Read the model definition and answer for the solid it produces. Units are mm, in the model's axes. A direction names the side the tool comes from. Round coordinates to 2 decimals unless told otherwise and drop trailing zeros. Write each loop counter-clockwise with the first axis right and the second up, starting at its lowest first coordinate (ties: lowest second). Pieces come first, ordered by that corner, then holes. Notation, with made-up numbers: (88, -23) - (122, -23) arc R13 cw to (122, -6) - close; hole circle Ø5 at (71, -34.5). An arc over 180 degrees is marked (long way). One line per item, written item: value. Start each with the question number.
(1) A cutting plane is placed at B-B, the plane y = 13. State how many separate pieces and enclosed holes the cut face has, plus the area to 3 significant figures.
(2) Find the intervals of material crossed by L1, parallel to X at y = 17.25, z = 0; L2, parallel to X at y = 14.25, z = -12; L3, parallel to Z at x = 24.5, y = 8, in increasing order.
(3) A cutting plane is placed at A-A, the plane z = 0. Determine the outline of the cut face in (x, y).
(4) The mould has two halves that part along Z. Classify faces 1 (the face through (-33.907, 11.619, 60.579)), 2 (the face through (-32.51, 11.62, -59.15)), 3 (the face through (35.41, 11, 1)): +Z half, -Z half, draft (parallel to the pull), parting line (faces both ways), or undercut.
(5) Flat-ended cylindrical pins translate along their axes: pin 1 Ø1.5 at (x, z) = (-6.5, 15) entering from +Y; pin 2 Ø8 at (x, y) = (19, 21.5) entering from +Z; pin 3 Ø8 at (x, z) = (0, 0) entering from +Y. Find the tip coordinate at first contact, or state that the pin passes through.
(6) For faces 4 (the face through (-35.41, 11, -1)), 5 (the face through (32.555, 11.619, -59.103)), determine the directions among +Z, -Z, +X, -X, +Y, -Y from which every point of the face is accessible in a straight line to the end or side of a thin tool.
(7) A cutting plane is placed at D-D, the plane x = 20.5. Determine the outline of the cut face in (y, z).
(8) A cutting plane is placed at C-C, the plane z = -44.5. Determine the outline of the cut face in (x, y), plus the area to 3 significant figures.
from build123d import *

# Parameters (mm, degrees)
BASE_EXTRUDE_DEPTH     = 20
FILLET1_R              = 5
FILLET2_R              = 3
SHELL1_T               = -2
RIB1_REACH             = 75.175
SKETCH6_WALLS_W        = 2
SKETCH6_WALLS_H        = 216.25372280356578
FILLET5_RADIUS         = 1
FILLET5_LENGTH         = 120.01036485
SKETCH3_R              = 10
CYLBOSS_DEPTH          = 25
FILLET4_R              = 1
COUNTERSNK_D           = 5
COUNTERSNK_CSINK_D     = 10
COUNTERSNK_CSINK_ANGLE = 90


with BuildPart() as part:
    # Sketch1 → Base-Extrude (new body)
    with BuildSketch(Plane(origin=(0, 0, 0), x_dir=(1, 0, 0), z_dir=(0, 1, 0))):
        Polygon((-35.41024463353893, -62.00518242476961), (35.410244633538916, -62.00518242476961), (35.41024463353893, 62.00518242476959), (-35.41024463353893, 62.00518242476961), align=None)
    extrude(amount=BASE_EXTRUDE_DEPTH)

    # Fillet1
    fillet1_edges = [part.edges().sort_by_distance(p)[0] for p in [
        (-35.41024463353893, 10, 62.00518242476961),
        (35.410244633538916, 10, 62.00518242476961),
        (35.41024463353893, 10, -62.00518242476959),
        (-35.41024463353893, 10, -62.00518242476961),
    ]]
    fillet(fillet1_edges, radius=FILLET1_R)

    # Fillet2
    fillet2_edges = [part.edges().sort_by_distance(p)[0] for p in [
        (-35.41024463353893, 0, 0),
        (0, 0, -62.0051824247696),
        (35.41024463353892, 0, 7.11e-15),
        (-7.11e-15, 0, 62.00518242476961),
        (33.94577853947167, 0, -60.54071633070233),
        (33.945778539471654, 0, 60.540716330702345),
        (-33.94577853947167, 0, 60.540716330702345),
        (-33.94577853947167, 0, -60.540716330702345),
    ]]
    fillet(fillet2_edges, radius=FILLET2_R)

    # Shell1
    shell1_openings = [part.faces().sort_by_distance(p)[0] for p in [
        (0, 20, 0),
    ]]
    offset(amount=SHELL1_T, openings=shell1_openings, kind=Kind.INTERSECTION)

    # Sketch6 walls → Rib1 (add, up to next)
    with BuildSketch(Plane(origin=(0, 16, 0), x_dir=(-1, 0, 0), z_dir=(0, 1, 0)), mode=Mode.PRIVATE) as rib1_sk1:
        with Locations((0, -0.4188286230260019)):
            Rectangle(SKETCH6_WALLS_W, SKETCH6_WALLS_H)
    rib1_tool1 = extrude(rib1_sk1.sketch, amount=-RIB1_REACH, mode=Mode.PRIVATE) - part.part
    add(rib1_tool1.solids().sort_by_distance((0, 16, -0.418828623))[0])

    # Fillet5: full round fillet: the end face becomes a half cylinder, R = half its width
    fillet5_face = Plane((0, 16, 0), x_dir=(0, 0, 1), z_dir=(0, 1, 0))  # on the end face: x along it, z out of the body
    fillet5_slab = fillet5_face.offset(-FILLET5_RADIUS / 2) * Box(FILLET5_LENGTH, 2 * FILLET5_RADIUS, FILLET5_RADIUS, mode=Mode.PRIVATE)  # the body's end, R deep
    fillet5_round = Plane((0, 15, 0), x_dir=(0, 1, 0), z_dir=(0, 0, 1)) * Cylinder(FILLET5_RADIUS, FILLET5_LENGTH, mode=Mode.PRIVATE)  # its axis R under the face
    add(fillet5_slab - fillet5_round, mode=Mode.SUBTRACT)

    # Sketch3 → CylBoss (add)
    with BuildSketch(Plane(origin=(0, 2, 0), x_dir=(-1, 0, 0), z_dir=(0, 1, 0))):
        with Locations(Location((0, 0, 0), (0, 0, 275.739170477))):
            Circle(SKETCH3_R)
    extrude(amount=CYLBOSS_DEPTH)

    # Fillet4
    fillet4_edges = [part.edges().sort_by_distance(p)[0] for p in [
        (1, 9, 60.00518242476961),
        (1, 9, -60.00518242476961),
        (-1, 9, 60.005182424769615),
        (-1, 9, -60.0051824247696),
        (-6e-17, 16, -60.005182425),
        (6e-17, 16, 60.005182425),
        (1, 2, -34.47752839791793),
        (1, 8.5, 9.9498743710662),
        (1, 8.5, -9.9498743710662),
        (-1, 2, -34.47752839792024),
        (-0.9999999999536726, 8.5, -9.949874371070855),
        (4.81118827973e-06, 15.999999999988425, -9.999999999998844),
        (-1, 8.5, 9.9498743710662),
        (-1, 8.5, 9.9498743710662),
        (-10, 2, -2.318834e-11),
        (10, 2, -1.8274e-13),
        (1, 2.292893218813452, 59.712289205956154),
        (-1, 2.292893218813452, 59.712289205956154),
        (1.0000000000000002, 2.292893218813452, -59.712289205956154),
        (-0.9999999999999999, 2.292893218813452, -59.712289205956154),
        (1, 2, 34.4775283979179),
        (-1, 2, 34.47752839791793),
    ]]
    fillet(fillet4_edges, radius=FILLET4_R)

    # CounterSnk (through all)
    with Locations(Plane(origin=(0, 27.000000000000004, 0), x_dir=(-1, 0, 0), z_dir=(0, 1, 0))):
        with Locations((0, 0)):
            CounterSinkHole(COUNTERSNK_D / 2, COUNTERSNK_CSINK_D / 2, counter_sink_angle=COUNTERSNK_CSINK_ANGLE)


solid = part.part
Here are the results:
1. separate pieces: 1
1. enclosed holes: 3
1. area: 1,250 mm²
2. L1: -35.41 to -33.41, -10 to -2.5, 2.5 to 10, 33.41 to 35.41
2. L2: -35.41 to -33.41, -1 to 1, 33.41 to 35.41
2. L3: -62.01 to -60.01, 60.01 to 62.01
3. outline: (-35.41, 3) arc R3 ccw to (-32.41, 0) - (-2.5, 0) - (-2.5, 24.5) - (-5, 27) - (-10, 27) - (-10, 3) arc R1 cw to (-11, 2) - (-32.41, 2) arc R1 cw to (-33.41, 3) - (-33.41, 20) - (-35.41, 20) - close; (2.5, 0) - (32.41, 0) arc R3 ccw to (35.41, 3) - (35.41, 20) - (33.41, 20) - (33.41, 3) arc R1 cw to (32.41, 2) - (11, 2) arc R1 cw to (10, 3) - (10, 27) - (5, 27) - (2.5, 24.5) - close
4. face 1: +Z half
4. face 2: undercut
4. face 3: draft
5. pin 1: y = 2
5. pin 2: z = 62.01
5. pin 3: y = 26
6. face 4: +Z, -Z, -X, +Y, -Y
6. face 5: +Y
7. outline: (0, -59.01) arc R3 ccw to (3, -62.01) - (20, -62.01) - (20, -60.01) - (3, -60.01) arc R1 cw to (2, -59.01) - (2, 59.01) arc R1 cw to (3, 60.01) - (20, 60.01) - (20, 62.01) - (3, 62.01) arc R3 ccw to (0, 59.01) - close
8. outline: (-35.41, 3) arc R3 ccw to (-32.41, 0) - (32.41, 0) arc R3 ccw to (35.41, 3) - (35.41, 20) - (33.41, 20) - (33.41, 3) arc R1 cw to (32.41, 2) - (2, 2) arc R1 cw to (1, 3) - (1, 15) arc R1 ccw to (-1, 15) - (-1, 3) arc R1 cw to (-2, 2) - (-32.41, 2) arc R1 cw to (-33.41, 3) - (-33.41, 20) - (-35.41, 20) - close
8. area: 238 mm²
